The listing builds one solid part. Answer for the finished solid, in the listing's coordinates (mm). A direction names the side the tool comes from. Round coordinates to 2 decimals unless told otherwise and drop trailing zeros. Write each loop counter-clockwise with the first axis right and the second up, starting at its lowest first coordinate (ties: lowest second). Pieces come first, ordered by that corner, then holes.
(1) For faces 1 (the face through (5.57, -3.16, -12.88)), 2 (the face through (0, -7, 17.069)), 3 (the face through (6, 3, 0)), determine the directions among +Z, -Z, +X, -X, +Y, -Y from which every point of the face is accessible in a straight line to the end or side of a thin tool.
(2) The mould has two halves that part along X. Classify faces 4 (the face through (0, 0, -26.492)), 5 (the face through (4.4, -4.8, -25.4)), 6 (the face through (5.522, 3.242, -12.878)), 7 (the face through (0.69, -3.1, -29.97)): +X half, -X half, draft (parallel to the pull), parting line (faces both ways), or undercut.
(3) Find the intervals of material crossed by probe 1 along Y at (x, z) = (0, -30) (3 decimals); probe 2 along Z at (x, y) = (7.25, -2.75); probe 3 along Z at (x, y) = (-5, 4), in increasing order.
(4) A cutting plane is placed at B-B, the plane z = 7.5. Give the vertices of the cut face in (x, y) (1 decimal).
(5) Each of these flat-tipped pins is pushed along its axis until it touches: pin 1 Ø1 at (y, z) = (-1.5, -4) entering from +X; pin 2 Ø1 at (y, z) = (1.5, 14) entering from -X; pin 3 Ø1.5 at (y, z) = (4, -9) entering from -X; pin 4 Ø5 at (x, y) = (-1, 1.5) entering from -Z. Where does it stop, or does it pass through?
from build123d import *

# Parameters (mm, degrees)
SKETCH2_OUTSIDE_W  = 30.382
SKETCH2_OUTSIDE_H  = 30.382
CUT_EXTRUDE1_DEPTH = 25.4
CHAMFER1_SIZE      = 0.508
SKETCH3_R          = 3.175
CUT_EXTRUDE2_DEPTH = 6.858
FILLET1_R          = 0.635


with BuildPart() as part:
    # Sketch1 → Revolve1 (revolve)
    with BuildSketch(Plane(origin=(0, 0, 0), x_dir=(0, 0, -1), z_dir=(1, 0, 0)), mode=Mode.PRIVATE) as revolve1_sk:
        Polygon((-25.019, 0), (-25.019, 6.35), (-17.0688, 6.35), (-17.0688, 7.9375), (0, 7.9375), (0, 7.62), (25.4, 7.62), (25.4, 6.35), (33.3502, 6.35), (33.3502, 0), align=None)
    revolve(revolve1_sk.sketch.rotate(Axis((0, 0, 0), (0, 0, 1)), 90), axis=Axis((0, 0, 0), (0, 0, 1)))

    # Sketch2 outside → Cut-Extrude1 (cut)
    with BuildSketch(Plane(origin=(0, 0, -25.4), x_dir=(-1, 0, 0), z_dir=(0, 0, -1))):
        Rectangle(SKETCH2_OUTSIDE_W, SKETCH2_OUTSIDE_H)
        Polygon((3.696970073, 6.40334), (-3.696970073, 6.40334), (-7.393940145, 0), (-3.696970073, -6.40334), (3.696970073, -6.40334), (7.393940145, 0), align=None, mode=Mode.SUBTRACT)
    extrude(amount=-CUT_EXTRUDE1_DEPTH, mode=Mode.SUBTRACT)

    # Chamfer1
    chamfer1_edges = [part.edges().sort_by_distance(p)[0] for p in [
        (6.35, 0, 25.019),
        (6.35, 0, -33.3502),
    ]]
    chamfer(chamfer1_edges, length=CHAMFER1_SIZE)

    # Sketch3 → Cut-Extrude2 (cut)
    with BuildSketch(Plane(origin=(0, 0, -33.3502), x_dir=(-1, 0, 0), z_dir=(0, 0, -1))):
        Circle(SKETCH3_R)
    extrude(amount=-CUT_EXTRUDE2_DEPTH, mode=Mode.SUBTRACT)

    # Fillet1
    fillet1_edges = [part.edges().sort_by_distance(p)[0] for p in [
        (-3.696970073, 6.40334, -12.7),
        (3.696970073, 6.40334, -12.7),
        (7.393940145, 0, -12.7),
        (3.696970073, -6.40334, -12.7),
        (-3.696970073, -6.40334, -12.7),
        (-7.393940145, 0, -12.7),
    ]]
    fillet(fillet1_edges, radius=FILLET1_R)


solid = part.part
Solutions:
1. face 1: -Z, +X, -Y
1. face 2: +Z
1. face 3: -Z
2. face 4: undercut
2. face 5: draft
2. face 6: +X half
2. face 7: undercut
3. probe 1: y = -6.35 to -3.175, 3.175 to 6.35
3. probe 2: z = 0 to 17.07
3. probe 3: z = -25.4 to 17.07
4. outline: circle Ø15.9 at (0, 0)
5. pin 1: stops at x = 6.82
5. pin 2: stops at x = -7.87
5. pin 3: stops at x = -5.52
5. pin 4: stops at z = -33.35
